The listing builds one solid part. Answer for the finished solid, in the listing's coordinates (mm). Round coordinates to 2 decimals unless told otherwise and drop trailing zeros. Write each loop counter-clockwise with the first axis right and the second up, starting at its lowest first coordinate (ties: lowest second). Pieces come first, ordered by that corner, then holes.
Item 1: Find section A-A on y = 0. Give the vertices of the cut face in (x, z).
Item 2: Find section C-C on z = 0.2. Give the vertices of the cut face in (x, y).
Item 3: Find the intervals of material crossed by probe 1 along Y at (x, z) = (60.25, 0.15); probe 2 along Y at (x, z) = (59.25, 0.3); probe 3 along X at (y, z) = (1, 0.15), in increasing order.
Item 4: Find section B-B on x = 59. Give the vertices of the cut face in (y, z).
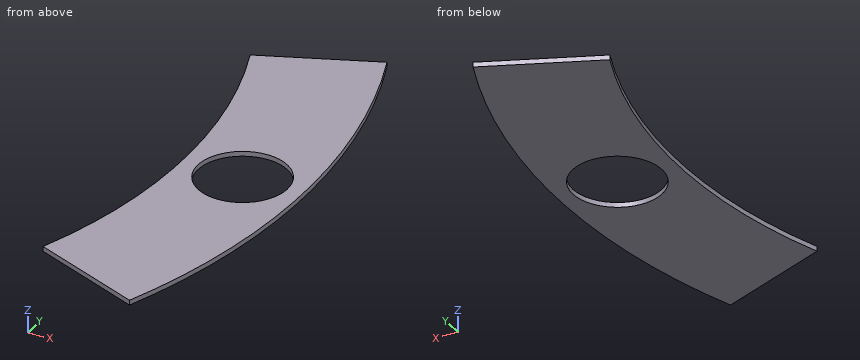
```python
from build123d import *

# Parameters (mm, degrees)
SKETCH4_R           = 68.072
BOSS_EXTRUDE2_DEPTH = 0.508
SKETCH5_R           = 55.372
CUT_EXTRUDE5_DEPTH  = 1.508
SKETCH6_R           = 4.699
CUT_EXTRUDE6_DEPTH  = 1.508
SKETCH8_OUTSIDE_W   = 176.652
SKETCH8_OUTSIDE_H   = 176.652
CUT_EXTRUDE11_DEPTH = 1.508


with BuildPart() as part:
    # Sketch4 → Boss-Extrude2 (new body)
    with BuildSketch(Plane.XY):
        Circle(SKETCH4_R)
    extrude(amount=BOSS_EXTRUDE2_DEPTH)

    # Sketch5 → Cut-Extrude5 (cut, through all)
    with BuildSketch(Plane.XY.offset(0.508)):
        Circle(SKETCH5_R)
    extrude(amount=-CUT_EXTRUDE5_DEPTH, mode=Mode.SUBTRACT)

    # Sketch6 → Cut-Extrude6 (cut, through all)
    with BuildSketch(Plane.XY.offset(0.508)):
        with Locations((61.722, 0)):
            Circle(SKETCH6_R)
    extrude(amount=-CUT_EXTRUDE6_DEPTH, mode=Mode.SUBTRACT)

    # Sketch8 outside → Cut-Extrude11 (cut, through all)
    with BuildSketch(Plane.XY.offset(0.508)):
        Rectangle(SKETCH8_OUTSIDE_W, SKETCH8_OUTSIDE_H)
        with BuildLine():
            Line((51.629608078, -20.011045792), (63.365389329, -24.872165551))
            ThreePointArc((63.365389329, -24.872165551), (68.072, 0), (63.365389329, 24.872165551))
            Line((63.365389329, 24.872165551), (51.629608078, 20.011045792))
            ThreePointArc((51.629608078, 20.011045792), (55.372, 0), (51.629608078, -20.011045792))
        make_face(mode=Mode.SUBTRACT)
    extrude(amount=-CUT_EXTRUDE11_DEPTH, mode=Mode.SUBTRACT)


solid = part.part
```
Check values:
1. outline: (55.37, 0) - (57.02, 0) - (57.02, 0.51) - (55.37, 0.51) - close; (66.42, 0) - (68.07, 0) - (68.07, 0.51) - (66.42, 0.51) - close
2. outline: (51.63, -20.01) - (63.37, -24.87) arc R68.07 ccw to (63.37, 24.87) - (51.63, 20.01) arc R55.37 cw to start; hole circle Ø9.4 at (61.72, 0)
3. probe 1: y = -23.58 to -4.46, 4.46 to 23.58
3. probe 2: y = -23.17 to -4, 4 to 23.17
3. probe 3: x = 55.36 to 57.13, 66.31 to 68.06
4. outline: (-23.06, 0) - (-3.83, 0) - (-3.83, 0.51) - (-23.06, 0.51) - close; (3.83, 0) - (23.06, 0) - (23.06, 0.51) - (3.83, 0.51) - close
